Geometry check sheet. Reference: the model listing, model coordinates, mm. Face numbers are marked on the shaded views. A direction names the side the tool comes from. Round coordinates to 2 decimals unless told otherwise and drop trailing zeros. Order: outer loops, then holes, each group sorted by start corner. A loop starts at its lowest first (then second) coordinate and runs counter-clockwise, first axis right, second up. Notation, with made-up numbers: (4.25, 50.5) -> (18.25, 50.5) arc R15 cw to (18.25, 75.5) -> close; hole circle Ø2 at (3.25, 41.25). An arc over 180 degrees is marked (long way). Use a Markdown table: item, result. Add a question column.
Item 1: Sectioned sample at B-B, the plane z = 5.75. Record the cut outline in (x, y), and give its area (3 significant figures).
Item 2: Sectioned sample at A-A, the plane z = 0. Record the cut outline in (x, y).
Item 3: Material ranges on probe 1 along Y at (x, z) = (5.75, -1.75); probe 2 along Y at (x, z) = (1.5, -2.75); probe 3 along Z at (x, y) = (-2, 1), recorded low to high. Write a range as [from, to].
Item 4: Mould release check, pull along Y, two halves, no side actions. Record for the marked faces 3, 4 and 5: pulls with the +Y half, pulls with the -Y half, needs draft (parallel to the pull), parting line crosses it, or undercut.
Item 5: Set-up check for the marked faces 1 and 2: record each of +Z, -Z, +X, -X, +Y, -Y from which the full face is reachable in a straight line by a thin tool's end or side.
Item 6: Gauge pin test, flat ends, axial feed: pin 1 Ø1.8 at (x, y) = (0, 10.16) entering from +Z; pin 2 Ø2 at (x, z) = (7, 5) entering from +Y; pin 3 Ø1 at (y, z) = (24.5, -2) entering from -X. Record the tip position at first contact, or that the pin passes through.
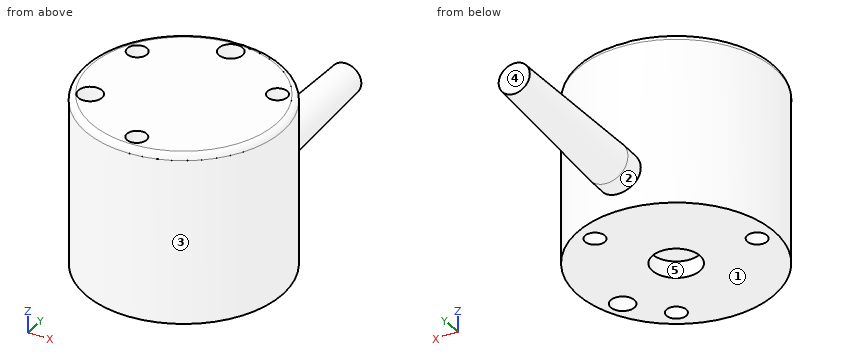
from build123d import *

# Parameters (mm, degrees)
BOSS_EXTRUDE1_DEPTH                 = 16.8
BOSS_EXTRUDE1_DEPTH_BACK            = 4.8
SKETCH1_R                           = 12.5
CIRPATTERN1_COUNT                   = 3
F_3_0MM_CLEARANCE_DOWEL_HOLE1_D     = 3
F_3_0MM_CLEARANCE_DOWEL_HOLE1_DEPTH = 3.3
F_3_0MM_CLEARANCE_DOWEL_HOLE1_TIP   = 0.901290929
CIRPATTERN2_COUNT                   = 3
F_3_0MM_CLEARANCE_DOWEL_HOLE2_D     = 3
F_3_0MM_CLEARANCE_DOWEL_HOLE2_DEPTH = 3.3
F_3_0MM_CLEARANCE_DOWEL_HOLE2_TIP   = 0.901290929
SKETCH10_R                          = 3.0175
CUT_EXTRUDE1_DEPTH                  = 2.1
FILLET1_R                           = 0.75
SKETCH11_R                          = 2.65
BOSS_EXTRUDE2_DEPTH                 = 15
SKETCH12_R                          = 2.65
BOSS_EXTRUDE3_DEPTH                 = 20
BOSS_EXTRUDE3_TAPER                 = 2


with BuildPart() as part:
    # Sketch1 → Boss-Extrude1 (new, two sides: drawn at the far end of the back side and taken through both)
    with BuildSketch(Plane.XY.offset(-BOSS_EXTRUDE1_DEPTH_BACK)):
        Circle(SKETCH1_R)
    extrude(amount=BOSS_EXTRUDE1_DEPTH + BOSS_EXTRUDE1_DEPTH_BACK)

    # Sketch2 → M3x0.5 Tapped Hole1 (revolve, cut)
    with BuildSketch(Plane(origin=(0, -10.16, 16.8), x_dir=(0, -1, 0), z_dir=(1, 0, 0))):
        Polygon((0, 0), (0, 8.251075774), (1.25, 7.5), (1.25, 0), align=None)
    m3x0_5_tapped_hole1 = revolve(axis=Axis((0, -10.16, 23.15), (0, 0, -1)), mode=Mode.SUBTRACT)

    # CirPattern1: M3x0.5 Tapped Hole1 ×3 about axis
    cirpattern1_axis = Axis((0, 0, 0), (0, 0, 1))
    for i in range(1, CIRPATTERN1_COUNT):
        add(m3x0_5_tapped_hole1.rotate(cirpattern1_axis, i * 360 / CIRPATTERN1_COUNT), mode=Mode.SUBTRACT)

    # 3.0mm Clearance Dowel Hole1
    with Locations(Plane.XY.offset(16.8)):
        with Locations((-8.799, -5.08), (0, 10.16)):
            Hole(F_3_0MM_CLEARANCE_DOWEL_HOLE1_D / 2, depth=F_3_0MM_CLEARANCE_DOWEL_HOLE1_DEPTH)
            with Locations((0, 0, -(F_3_0MM_CLEARANCE_DOWEL_HOLE1_DEPTH + F_3_0MM_CLEARANCE_DOWEL_HOLE1_TIP / 2))):  # 118° drill point
                Cone(0, F_3_0MM_CLEARANCE_DOWEL_HOLE1_D / 2, F_3_0MM_CLEARANCE_DOWEL_HOLE1_TIP, mode=Mode.SUBTRACT)

    # Sketch6 → M3x0.5 Tapped Hole2 (revolve, cut)
    with BuildSketch(Plane(origin=(-10.16, 0, -4.8), x_dir=(0, 1, 0), z_dir=(1, 0, 0))):
        Polygon((0, 0), (0, 8.251075774), (1.25, 7.5), (1.25, 0), align=None)
    m3x0_5_tapped_hole2 = revolve(axis=Axis((-10.16, 0, -11.15), (0, 0, 1)), mode=Mode.SUBTRACT)

    # CirPattern2: M3x0.5 Tapped Hole2 ×3 about axis
    cirpattern2_axis = Axis((0, 0, 0), (0, 0, 1))
    for i in range(1, CIRPATTERN2_COUNT):
        add(m3x0_5_tapped_hole2.rotate(cirpattern2_axis, i * 360 / CIRPATTERN2_COUNT), mode=Mode.SUBTRACT)

    # 3.0mm Clearance Dowel Hole2
    with Locations(Plane(origin=(0, 0, -4.8), x_dir=(-1, 0, 0), z_dir=(0, 0, -1))):
        with Locations((-9.208, -4.294)):
            Hole(F_3_0MM_CLEARANCE_DOWEL_HOLE2_D / 2, depth=F_3_0MM_CLEARANCE_DOWEL_HOLE2_DEPTH)
            with Locations((0, 0, -(F_3_0MM_CLEARANCE_DOWEL_HOLE2_DEPTH + F_3_0MM_CLEARANCE_DOWEL_HOLE2_TIP / 2))):  # 118° drill point
                Cone(0, F_3_0MM_CLEARANCE_DOWEL_HOLE2_D / 2, F_3_0MM_CLEARANCE_DOWEL_HOLE2_TIP, mode=Mode.SUBTRACT)

    # Sketch10 → Cut-Extrude1 (cut)
    with BuildSketch(Plane(origin=(0, 0, -4.8), x_dir=(-1, 0, 0), z_dir=(0, 0, -1))):
        Circle(SKETCH10_R)
    extrude(amount=-CUT_EXTRUDE1_DEPTH, mode=Mode.SUBTRACT)

    # Fillet1
    fillet1_edges = [part.edges().sort_by_distance(p)[0] for p in [
        (-12.5, 0, 16.8),
    ]]
    fillet(fillet1_edges, radius=FILLET1_R)

    # Sketch11 → Boss-Extrude2 (add)
    with BuildSketch(Plane(origin=(0, 0, 0), x_dir=(1, 0, 0), z_dir=(0, 1, 0))):
        with Locations(Location((0, 0, 0), (0, 0, 90))):
            Circle(SKETCH11_R)
    extrude(amount=BOSS_EXTRUDE2_DEPTH)

    # Sketch12 → Boss-Extrude3 (add)
    with BuildSketch(Plane(origin=(0, 15, 0), x_dir=(1, 0, 0), z_dir=(0, 1, 0))):
        with Locations(Location((0, 0, 0), (0, 0, 90))):
            Circle(SKETCH12_R)
    extrude(amount=BOSS_EXTRUDE3_DEPTH, taper=BOSS_EXTRUDE3_TAPER)


solid = part.part
Found:
| question | item | result |
|---|---|---|
| 1 | outline | circle Ø25 at (0, 0) |
| 1 | area | 491 mm2 |
| 2 | outline | (-2.65, 12.22) arc R12.5 ccw (long way) to (2.65, 12.22) -> (2.65, 15) -> (1.95, 35) -> (-1.95, 35) -> (-2.65, 15) -> close; hole circle Ø2.5 at (-10.16, 0); hole circle Ø2.5 at (5.08, -8.8); hole circle Ø2.5 at (5.08, 8.8) |
| 3 | probe 1 | y = [-11.1, -9.85], [-7.74, 7.74], [9.85, 11.1] |
| 3 | probe 2 | y = [-12.41, -2.62], [2.62, 12.41] |
| 3 | probe 3 | z = [-2.7, 16.8] |
| 4 | face 3 | parting line crosses it |
| 4 | face 4 | pulls with the +Y half |
| 4 | face 5 | undercut |
| 5 | face 1 | -Z, +X, -X, +Y, -Y |
| 5 | face 2 | +Y |
| 6 | pin 1 | stops at z = 13.14 |
| 6 | pin 2 | stops at y = 10.97 |
| 6 | pin 3 | stops at x = -1.77 |
